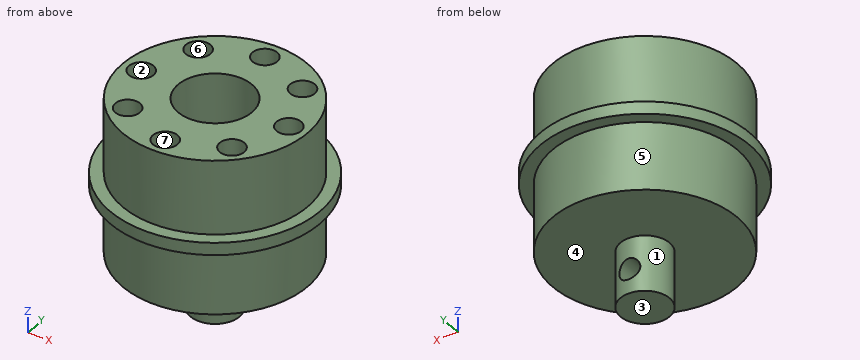
```python
from build123d import *

# Parameters (mm, degrees)
SKETCH_1_R                    = 17
EXTRUDE_1_DEPTH               = 25
SKETCH_3_R                    = 4
EXTRUDE_3_DEPTH               = 9
SKETCH_4_R                    = 17
SKETCH_4_R_2                  = 15
CUT_EXTRUDE_1_DEPTH           = 11
CUT_EXTRUDE_START             = -12
SKETCH_5_R                    = 17
SKETCH_5_R_2                  = 15
CUT_EXTRUDE_2_DEPTH           = 12
HOLE_WIZARD_M4_1_D            = 3.3
HOLE_WIZARD_M4_1_DEPTH        = 10.1
HOLE_WIZARD_M4_1_CBORE_D      = 4
HOLE_WIZARD_M4_1_CBORE_DEPTH  = 8
HOLE_WIZARD_M4_1_TIP          = 0.991420021
CUT_EXTRUDE_3_DEPTH           = 10
CUT_EXTRUDE_3_DEPTH_BACK      = 10
SKETCH_9_R                    = 1.7
HOLE_WIZARD_M12_1_D           = 10.2
HOLE_WIZARD_M12_1_DEPTH       = 19.25
HOLE_WIZARD_M12_1_CBORE_D     = 12
HOLE_WIZARD_M12_1_CBORE_DEPTH = 14
HOLE_WIZARD_M12_1_TIP         = 3.064389157


with BuildPart() as part:
    # Sketch 1 → Extrude 1 (new body)
    with BuildSketch(Plane.XY):
        Circle(SKETCH_1_R)
    extrude(amount=EXTRUDE_1_DEPTH)

    # Sketch 3 → Extrude 3 (add)
    with BuildSketch(Plane(origin=(0, 0, 0), x_dir=(-1, 0, 0), z_dir=(0, 0, -1))):
        with Locations(Location((0, 0, 0), (0, 0, 180))):
            Circle(SKETCH_3_R)
    extrude(amount=EXTRUDE_3_DEPTH)

    # Sketch 4 → Cut-Extrude 1 (cut)
    with BuildSketch(Plane(origin=(0, 0, 0), x_dir=(-1, 0, 0), z_dir=(0, 0, -1))):
        Circle(SKETCH_4_R)
        Circle(SKETCH_4_R_2, mode=Mode.SUBTRACT)
    extrude(amount=-CUT_EXTRUDE_1_DEPTH, mode=Mode.SUBTRACT)

    # Sketch 5 → Cut-Extrude 2 (cut)
    with BuildSketch(Plane.XY.offset(25).offset(CUT_EXTRUDE_START)):
        with Locations(Location((0, 0, 0), (0, 0, 180))):
            Circle(SKETCH_5_R)
        with Locations(Location((0, 0, 0), (0, 0, 180))):
            Circle(SKETCH_5_R_2, mode=Mode.SUBTRACT)
    extrude(amount=CUT_EXTRUDE_2_DEPTH, mode=Mode.SUBTRACT)

    # Hole Wizard M4 _1
    with Locations(Plane(origin=(-12, 0, 25), x_dir=(1, 0, 0), z_dir=(0, 0, 1))):
        with Locations((0, 0), (3.514718626, 8.485281374), (12, 12), (20.485281374, 8.485281374), (24, 0), (20.485281374, -8.485281374), (3.514718626, -8.485281374), (12, -12)):
            CounterBoreHole(HOLE_WIZARD_M4_1_D / 2, HOLE_WIZARD_M4_1_CBORE_D / 2, HOLE_WIZARD_M4_1_CBORE_DEPTH, depth=HOLE_WIZARD_M4_1_DEPTH)
            with Locations((0, 0, -(HOLE_WIZARD_M4_1_DEPTH + HOLE_WIZARD_M4_1_TIP / 2))):  # 118° drill point
                Cone(0, HOLE_WIZARD_M4_1_D / 2, HOLE_WIZARD_M4_1_TIP, mode=Mode.SUBTRACT)

    # Sketch 9 → Cut-Extrude 3 (cut, two sides: drawn at the far end of the back side and taken through both)
    with BuildSketch(Plane(origin=(0, 0, 0), x_dir=(1, 0, 0), z_dir=(0, 1, 0)).offset(-CUT_EXTRUDE_3_DEPTH_BACK)):
        with Locations(Location((0, 5, 0), (0, 0, 270))):
            Circle(SKETCH_9_R)
    extrude(amount=CUT_EXTRUDE_3_DEPTH + CUT_EXTRUDE_3_DEPTH_BACK, mode=Mode.SUBTRACT)

    # Hole Wizard M12 _1
    with Locations(Plane.XY.offset(25)):
        with Locations((0, 0)):
            CounterBoreHole(HOLE_WIZARD_M12_1_D / 2, HOLE_WIZARD_M12_1_CBORE_D / 2, HOLE_WIZARD_M12_1_CBORE_DEPTH, depth=HOLE_WIZARD_M12_1_DEPTH)
            with Locations((0, 0, -(HOLE_WIZARD_M12_1_DEPTH + HOLE_WIZARD_M12_1_TIP / 2))):  # 118° drill point
                Cone(0, HOLE_WIZARD_M12_1_D / 2, HOLE_WIZARD_M12_1_TIP, mode=Mode.SUBTRACT)


solid = part.part
```
Geometry check sheet. Reference: the model listing, model coordinates, mm. Face numbers are marked on the shaded views. A direction names the side the tool comes from. Coordinates: 2 decimals unless noted, no trailing zeros. Loops run counter-clockwise (first coordinate to the right, second up) from the corner with the lowest first, then second, coordinate; pieces in that order, holes last.
Item 1: Access from +Z, -Z, +X, -X, +Y, -Y to the whole of each face (thin tool, end or side, straight path). Record for the marked faces 1, 2 and 3.
Item 2: Sectioned sample at A-A, the plane z = 6.5. Record the boundary of the cut face in (x, y).
Item 3: Thickness scan on line 1 (X direction, y = 7.5, z = 22.5); line 2 (X direction, y = -7.5, z = 15). Record the ranges inside material, lowest first.
Item 4: Sectioned sample at C-C, the plane z = 18.5. Count the separate pieces of the cut face and the enclosed holes in it, then the cut area to 3 significant figures.
Item 5: Go/stop test with flat-tipped pins: pin 1 Ø4 at (y, z) = (-9.5, 16) entering from +X; pin 2 Ø1.2 at (x, y) = (7.5, 8.5) entering from +Z; pin 3 Ø2 at (x, z) = (8.5, 20) entering from +Y. Record where each tip stops, or that it passes through.
Item 6: Release check for a two-part mould opening along X. For the marked faces 4, 5, 6 and 7 record: released by +X, released by -X, zero draft, split by the parting line, or undercut.
Item 7: Sectioned sample at D-D, the plane z = -5. Record the boundary of the cut face in (x, y).
Item 8: Sectioned sample at B-B, the plane y = 14.5. Record the boundary of the cut face in (x, z).
Check result:
1. face 1: -Z
1. face 2: +Z
1. face 3: -Z, +X, -X, +Y, -Y
2. outline: circle Ø30 at (0, 0); hole circle Ø10.2 at (0, 0)
3. line 1: x = -12.99 to -10.23, -6.74 to 6.74, 10.23 to 12.99
3. line 2: x = -12.99 to -9.81, -7.16 to 7.16, 9.81 to 12.99
4. separate pieces: 1
4. enclosed holes: 9
4. area: 493 mm2
5. pin 1: stops at x = 12.99
5. pin 2: stops at z = 14.86
5. pin 3: stops at y = 12.99
6. face 4: zero draft
6. face 5: split by the parting line
6. face 6: undercut
6. face 7: undercut
7. outline: (-1.7, -3.62) - (-1.7, 3.62) arc R4 ccw to start; (1.7, -3.62) arc R4 ccw to (1.7, 3.62) - close
8. outline: (-8.87, 11) - (-3.84, 11) - (-3.84, 0) - (3.84, 0) - (3.84, 11) - (8.87, 11) - (8.87, 13) - (3.84, 13) - (3.84, 25) - (-3.84, 25) - (-3.84, 13) - (-8.87, 13) - close
